Geometry check sheet. Reference: the model listing, model coordinates, mm. Round coordinates to 2 decimals unless told otherwise and drop trailing zeros. Loops run counter-clockwise (first coordinate to the right, second up) from the corner with the lowest first, then second, coordinate; pieces in that order, holes last. Notation, with made-up numbers: (-32.5, 69.5) - (25.5, 69.5) arc R14 ccw to (25.5, 95.5) - close; hole circle Ø4 at (65, 30.25). An arc over 180 degrees is marked (long way). Write item = value, one per line.
```python
from build123d import *

# Parameters (mm, degrees)
ESQUISSE1_W             = 100
ESQUISSE1_H             = 65
BOSS_EXTRU_1_DEPTH      = 5
ESQUISSE2_W             = 15
ESQUISSE2_H             = 5.01
ESQUISSE2_W_2           = 15.01
ESQUISSE2_W_3           = 14.51
ESQUISSE2_W_4           = 5
ESQUISSE2_H_2           = 17.5
ENL_V_MAT_EXTRU_1_DEPTH = 5
ESQUISSE3_R             = 9.505
ENL_V_MAT_EXTRU_2_DEPTH = 10
ENL_V_MAT_EXTRU_3_DEPTH = 10


with BuildPart() as part:
    # Esquisse1 → Boss.-Extru.1 (new body)
    with BuildSketch(Plane.XY):
        Rectangle(ESQUISSE1_W, ESQUISSE1_H)
    extrude(amount=BOSS_EXTRU_1_DEPTH)

    # Esquisse2 → Enlèv. mat.-Extru.1 (cut)
    with BuildSketch(Plane.XY.offset(5)):
        with Locations((-42.5, 29.995)):
            Rectangle(ESQUISSE2_W, ESQUISSE2_H)
        with Locations((-14.005, 29.995)):
            Rectangle(ESQUISSE2_W_2, ESQUISSE2_H)
        with Locations((14.495, 29.995)):
            Rectangle(ESQUISSE2_W_2, ESQUISSE2_H)
        with Locations((42.745, 30.005)):
            Rectangle(ESQUISSE2_W_3, ESQUISSE2_H)
        with Locations((-47.5, 0.25)):
            Rectangle(ESQUISSE2_W_4, ESQUISSE2_H_2)
        with Locations((47.5, 0.25)):
            Rectangle(ESQUISSE2_W_4, ESQUISSE2_H_2)
        with Locations((42.745, -30.005)):
            Rectangle(ESQUISSE2_W_3, ESQUISSE2_H)
        with Locations((14.495, -29.995)):
            Rectangle(ESQUISSE2_W_2, ESQUISSE2_H)
        with Locations((-14.005, -29.995)):
            Rectangle(ESQUISSE2_W_2, ESQUISSE2_H)
        with Locations((-42.5, -29.995)):
            Rectangle(ESQUISSE2_W, ESQUISSE2_H)
    extrude(amount=-ENL_V_MAT_EXTRU_1_DEPTH, mode=Mode.SUBTRACT)

    # Esquisse3 → Enlèv. mat.-Extru.2 (cut)
    with BuildSketch(Plane.XY.offset(5)):
        with Locations((-12, -13)):
            Circle(ESQUISSE3_R)
    extrude(amount=-ENL_V_MAT_EXTRU_2_DEPTH, mode=Mode.SUBTRACT)

    # Esquisse4 → Enlèv. mat.-Extru.3 (cut)
    with BuildSketch(Plane.XY.offset(5)):
        with BuildLine():
            Line((24.445837429, 0.203360159), (19.045949486, -2.412210563))
            ThreePointArc((19.045949486, -2.412210563), (13.695630827, -0.553678818), (15.554162571, 4.796639841))
            Line((15.554162571, 4.796639841), (20.954050514, 7.412210563))
            ThreePointArc((20.954050514, 7.412210563), (26.304369173, 5.553678818), (24.445837429, 0.203360159))
        make_face()
    extrude(amount=-ENL_V_MAT_EXTRU_3_DEPTH, mode=Mode.SUBTRACT)


solid = part.part
```
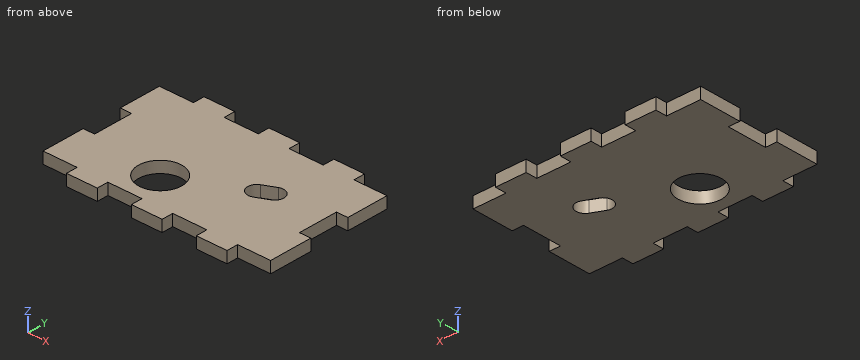
(1) Section check A-A (y = -13). Enter the section's corners in (x, z) (3 decimals), then the cut area to 3 significant figures.
Answers follow:
outline = (-50, 0) - (-21.505, 0) - (-21.505, 5) - (-50, 5) - close; (-2.495, 0) - (50, 0) - (50, 5) - (-2.495, 5) - close
area = 405 mm²
(2) Section check C-C (z = 3.9). State how many separate pieces and enclosed holes the cut face has, then the cut area to 3 significant figures.
Answers follow:
separate_pieces = 1
enclosed_holes = 2
area = 5,350 mm²
(3) Gauge pin test, flat ends, axial feed: pin 1 (1.5 mm diameter, centred on x = 11.5, z = 2.5, fed in from -Y); pin 2 (1.5 mm diameter, centred on x = 45, z = 1.5, fed in from +Y); pin 3 (1.5 mm diameter, centred on y = -31, z = 2.5, fed in from +X). Record the tip position at first contact, or that the pin passes through.
Answers follow:
pin_1 = -27.49
pin_2 = 27.5
pin_3 = 35.49
(4) Section check B-B (x = -5). Enter the section's corners in (y, z), then the cut area to 3 significant figures.
Answers follow:
outline = (-32.5, 0) - (-19.43, 0) - (-19.43, 5) - (-32.5, 5) - close; (-6.57, 0) - (32.5, 0) - (32.5, 5) - (-6.57, 5) - close
area = 261 mm²
(5) Scan lines: L1, parallel to X at y = 30, z = 0.8; L2, parallel to Y at x = -12, z = 2.35 (3 decimals); L3, parallel to X at y = 1, z = 1.3. Record each from-to range of solid material in increasing order. Write a range as [from, to].
Answers follow:
L1 = [-35, -21.51], [-6.5, 6.99], [22, 35.49]
L2 = [-27.49, -22.505], [-3.495, 27.49]
L3 = [-45, 13.3], [25.56, 45]
